Geometry: final body of the model. Coordinates: model frame, mm. A direction names the side the tool comes from. Round coordinates to 2 decimals unless told otherwise and drop trailing zeros. Loops run counter-clockwise (first coordinate to the right, second up) from the corner with the lowest first, then second, coordinate; pieces in that order, holes last. Notation, with made-up numbers: (21.25, -28.5) - (56.25, -28.5) arc R24 cw to (56.25, -10.5) - close; hole circle Ø7 at (32.25, 45). An arc over 180 degrees is marked (long way). Answer in a Markdown table with one row per item. Add a question column.
from build123d import *

# Parameters (mm, degrees)
F0_W     = 374.65
F0_H     = 76.2
F1_DEPTH = 22.225
F2_W     = 34.925
F2_H     = 6.35
F3_DEPTH = 76.2
F4_W     = 9.525
F4_H     = 9.525
F5_DEPTH = 374.65


with BuildPart() as f1:
    # F0 (on Front) → F1 (new body)
    with BuildSketch(Plane.XZ):
        with Locations((187.325, 38.1)):
            Rectangle(F0_W, F0_H)
    extrude(amount=F1_DEPTH)

    # F2 (on face) → F3 (cut, through all)
    with BuildSketch(Plane.XY.offset(76.2)):
        with Locations((17.4625, -3.175)):
            Rectangle(F2_W, F2_H)
        with Locations((17.4625, -19.05)):
            Rectangle(F2_W, F2_H)
        with Locations((357.1875, -3.175)):
            Rectangle(F2_W, F2_H)
        with Locations((357.1875, -19.05)):
            Rectangle(F2_W, F2_H)
    extrude(amount=-F3_DEPTH, mode=Mode.SUBTRACT)

    # F4 (on face) → F5 (cut, through all)
    with BuildSketch(Plane(origin=(0, 0, 0), x_dir=(0, -1, 0), z_dir=(-1, 0, 0))):
        with Locations((11.1125, 71.4375)):
            Rectangle(F4_W, F4_H)
        with Locations((11.1125, 4.7625)):
            Rectangle(F4_W, F4_H)
    extrude(amount=-F5_DEPTH, mode=Mode.SUBTRACT)


solid = f1.part
1) Pull-direction query (Y, two-part tool) for faces 1 (the flat face through (185, -3, 0)), 2 (the flat face through (357, -15.875, 39)), 3 (the flat face through (185, -6.35, 5)), 4 (the flat face through (185, -11, 9.525)); classes: pulls with the +Y half, pulls with the -Y half, needs draft (parallel to the pull), parting line crosses it, or undercut.
2) Material intervals for line 1 along Y through (x, z) = (214.5, 68) (3 decimals); line 2 along Y through (x, z) = (26.5, 48) (3 decimals); line 3 along Z through (x, y) = (352, -11.5) (3 decimals), sorted ascending. Write a range as from..to.
3) Section B-B, the plane z = 14. Return the cut outline in (x, y) (3 decimals).
4) Reachability of faces 5 (the flat face through (34.925, -3, 39)), 6 (the flat face through (34.925, -19, 39)), 7 (the flat face through (357, -6.35, 39)) from +Z, -Z, +X, -X, +Y, -Y: full face, straight path, thin tool, end or side. Return the list, or none.
5) Section C-C, the plane x = 29.5. Return the cut outline in (y, z) (3 decimals), and give its area (3 significant figures).
6) Section A-A, the plane x = 304.5. Return the cut outline in (y, z) (3 decimals).
7) Contact query for flat-ended pins moving along their axis: pin 1 Ø10.5 at (x, z) = (22, 39) entering from +Y; pin 2 Ø5 at (y, z) = (-18.5, 37.5) entering from -X (3 decimals); pin 3 Ø1.9 at (y, z) = (-3, 52) entering from +X (3 decimals). Output: stop coordinate, or through.
Evaluation:
| question | item | result |
|---|---|---|
| 1 | face 1 | needs draft |
| 1 | face 2 | pulls with the -Y half |
| 1 | face 3 | undercut |
| 1 | face 4 | undercut |
| 2 | line 1 | y = -22.225..-15.875, -6.35..0 |
| 2 | line 2 | y = -15.875..-6.35 |
| 2 | line 3 | z = 9.525..66.675 |
| 3 | outline | (0, -15.875) - (34.925, -15.875) - (34.925, -22.225) - (339.725, -22.225) - (339.725, -15.875) - (374.65, -15.875) - (374.65, -6.35) - (339.725, -6.35) - (339.725, 0) - (34.925, 0) - (34.925, -6.35) - (0, -6.35) - close |
| 4 | face 5 | +Z, -Z, -X, +Y |
| 4 | face 6 | +Z, -Z, -X, -Y |
| 4 | face 7 | +Z, -Z, +X, +Y |
| 5 | outline | (-15.875, 9.525) - (-6.35, 9.525) - (-6.35, 66.675) - (-15.875, 66.675) - close |
| 5 | area | 544 mm² |
| 6 | outline | (-22.225, 0) - (-15.875, 0) - (-15.875, 9.525) - (-6.35, 9.525) - (-6.35, 0) - (0, 0) - (0, 76.2) - (-6.35, 76.2) - (-6.35, 66.675) - (-15.875, 66.675) - (-15.875, 76.2) - (-22.225, 76.2) - close |
| 7 | pin 1 | stops at y = -6.35 |
| 7 | pin 2 | stops at x = 34.925 |
| 7 | pin 3 | stops at x = 339.725 |
